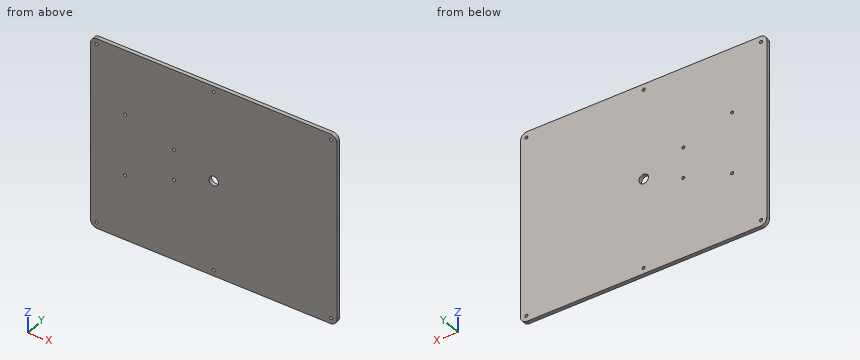
```python
from build123d import *

# Parameters (mm, degrees)
CROQUIS1_R              = 4
SALIENTE_EXTRUIR1_DEPTH = 10
CROQUIS2_R              = 4
CROQUIS2_R_2            = 12.5
CORTAR_EXTRUIR1_DEPTH   = 10


with BuildPart() as part:
    # Croquis1 → Saliente-Extruir1 (new body)
    with BuildSketch(Plane(origin=(0, 0, 0), x_dir=(1, 0, 0), z_dir=(0, 1, 0))):
        with BuildLine():
            Line((-303, 250), (303, 250))
            ThreePointArc((303, 250), (315.02081528, 245.02081528), (320, 233))
            Line((320, 233), (320, -233))
            ThreePointArc((320, -233), (315.02081528, -245.02081528), (303, -250))
            Line((303, -250), (-303, -250))
            ThreePointArc((-303, -250), (-315.02081528, -245.02081528), (-320, -233))
            Line((-320, -233), (-320, 233))
            ThreePointArc((-320, 233), (-315.02081528, 245.02081528), (-303, 250))
        make_face()
        with Locations((0, 235)):
            Circle(CROQUIS1_R, mode=Mode.SUBTRACT)
        with Locations((305, 235)):
            Circle(CROQUIS1_R, mode=Mode.SUBTRACT)
        with Locations((-305, 235)):
            Circle(CROQUIS1_R, mode=Mode.SUBTRACT)
        with Locations((0, -235)):
            Circle(CROQUIS1_R, mode=Mode.SUBTRACT)
        with Locations((305, -235)):
            Circle(CROQUIS1_R, mode=Mode.SUBTRACT)
        with Locations((-305, -235)):
            Circle(CROQUIS1_R, mode=Mode.SUBTRACT)
    extrude(amount=SALIENTE_EXTRUIR1_DEPTH)

    # Croquis2 → Cortar-Extruir1 (cut)
    with BuildSketch(Plane(origin=(0, 10, 0), x_dir=(1, 0, 0), z_dir=(0, 1, 0))):
        with Locations((-230, 80)):
            Circle(CROQUIS2_R)
        with Locations((-103, 40)):
            Circle(CROQUIS2_R)
        Circle(CROQUIS2_R_2)
        with Locations((-103, -40)):
            Circle(CROQUIS2_R)
        with Locations((-230, -80)):
            Circle(CROQUIS2_R)
    extrude(amount=-CORTAR_EXTRUIR1_DEPTH, mode=Mode.SUBTRACT)


solid = part.part
```
For this review, take the finished solid that the model builds, in its own axes (mm). Coordinates: 2 decimals unless noted, no trailing zeros. Write each loop counter-clockwise with the first axis right and the second up, starting at its lowest first coordinate (ties: lowest second). Pieces come first, ordered by that corner, then holes. Notation, with made-up numbers: (78, 12) - (117, 12) arc R28 ccw to (117, 47) - close; hole circle Ø5 at (-3, 68). An arc over 180 degrees is marked (long way). Answer in a Markdown table with one row per item. Add a question column.
Q1. We need section A-A, the plane z = 0. State the section outline as (x, y) points, and give its area (3 significant figures).
Q2. For probe 1 along X at (y, z) = (6.25, 235); probe 2 along Z at (x, y) = (-103, 5.75); probe 3 along X at (y, z) = (8.5, -80), list the stretches that pass through material, from the lowest coordinate up.
Q3. For P1, Ø5, axis at x = 305, z = -235, coming from the +Y side, flat-tipped, find the tip position at first contact; note if it passes through.
Answer list:
| question | item | result |
|---|---|---|
| 1 | outline | (-320, 0) - (-12.5, 0) - (-12.5, 10) - (-320, 10) - close; (12.5, 0) - (320, 0) - (320, 10) - (12.5, 10) - close |
| 1 | area | 6,150 mm2 |
| 2 | probe 1 | x = -319.88 to -309, -301 to -4, 4 to 301, 309 to 319.88 |
| 2 | probe 2 | z = -250 to -44, -36 to 36, 44 to 250 |
| 2 | probe 3 | x = -320 to -234, -226 to 320 |
| 3 | P1 | passes through |
